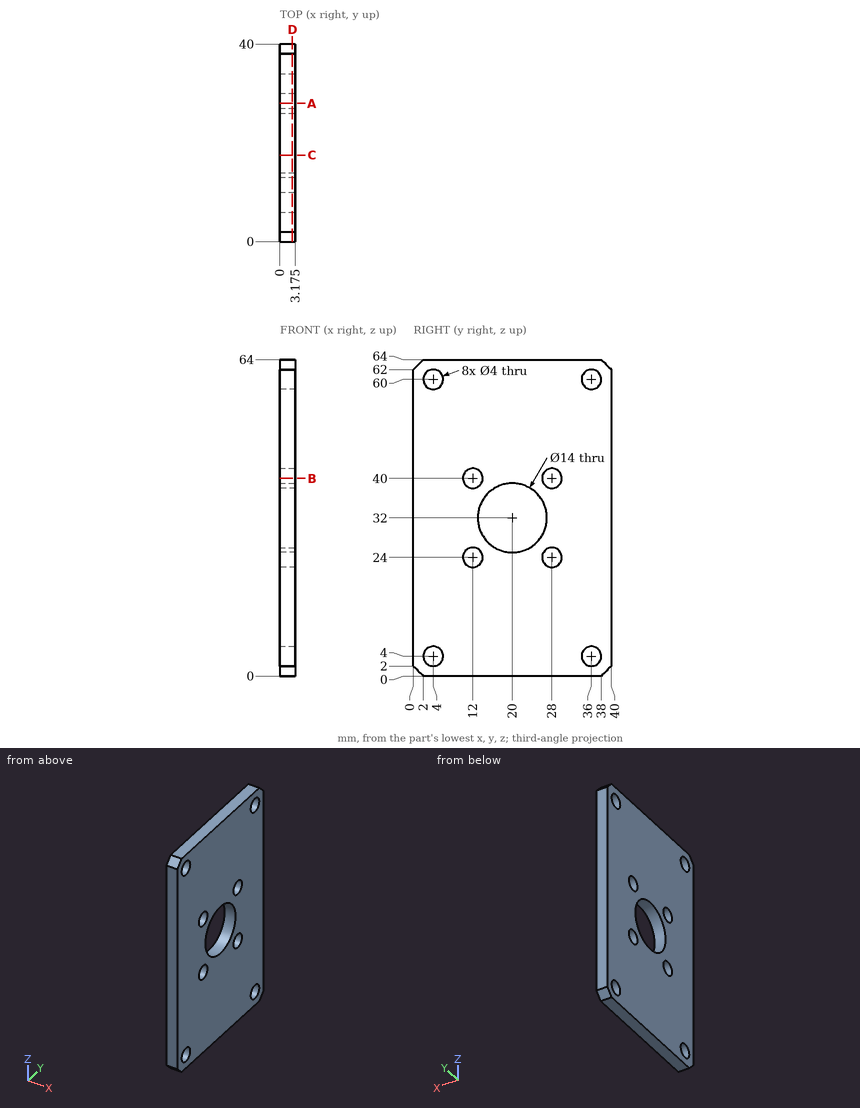
Input: dimensioned drawing with shaded views. Units: mm. Origin: part minimum x, y, z. Give positions to 0.01 mm unless a question says otherwise; leave off trailing zeros. Order: outer loops, then holes, each group sorted by start corner. A loop starts at its lowest first (then second) coordinate and runs counter-clockwise, first axis right, second up.
(1) Section query C-C (y = 17.5). Return the cut outline in (x, z) (3 decimals), plus the area to 3 significant figures.
(2) Section query B-B (z = 40). Return the cut outline in (x, y) (3 decimals), plus the area to 3 significant figures.
(3) Section query A-A (y = 28). Return the cut outline in (x, z) (3 decimals), plus the area to 3 significant figures.
(4) Section query D-D (x = 2.55). State how many separate pieces and enclosed holes the cut face has, plus the area to 3 significant figures.
(5) Contact query for a flat-ended pin moving along its axis: P1, Ø18, axis at y = 20, z = 32, coming from the +X side (3 decimals). Output: stop coordinate, or through.
(6) Material intervals for line 1 along Y through (x, z) = (0.75, 60); line 2 along Y through (x, z) = (1.7, 40); line 3 along Z through (x, y) = (1.3, 36.5), sorted ascending.
Outcome:
1. outline: (0, 0) - (3.175, 0) - (3.175, 25.462) - (0, 25.462) - close; (0, 38.538) - (3.175, 38.538) - (3.175, 64) - (0, 64) - close
1. area: 162 mm2
2. outline: (0, 0) - (3.175, 0) - (3.175, 10) - (0, 10) - close; (0, 14) - (3.175, 14) - (3.175, 26) - (0, 26) - close; (0, 30) - (3.175, 30) - (3.175, 40) - (0, 40) - close
2. area: 102 mm2
3. outline: (0, 0) - (3.175, 0) - (3.175, 22) - (0, 22) - close; (0, 26) - (3.175, 26) - (3.175, 38) - (0, 38) - close; (0, 42) - (3.175, 42) - (3.175, 64) - (0, 64) - close
3. area: 178 mm2
4. separate pieces: 1
4. enclosed holes: 9
4. area: 2,300 mm2
5. P1: stops at x = 3.175
6. line 1: y = 0 to 2, 6 to 34, 38 to 40
6. line 2: y = 0 to 10, 14 to 26, 30 to 40
6. line 3: z = 0 to 2.06, 5.94 to 58.06, 61.94 to 64
